CAD build for the part. Positions are in the model's coordinates, mm. A direction names the side the tool comes from. Give positions to 0.01 mm unless a question says otherwise; leave off trailing zeros. Loops run counter-clockwise (first coordinate to the right, second up) from the corner with the lowest first, then second, coordinate; pieces in that order, holes last. Notation, with made-up numbers: M 20.5,71.25 L 76.5,71.25 A20 ccw 76.5,94.25 Z; hole C 30,48.25 d1. An arc over 180 degrees is marked long. Answer as CSV lines item,"result".
```python
from build123d import *

# Parameters (mm, degrees)
BOSS_EXTRUDE1_DEPTH = 7
SKETCH2_R           = 5
CUT_EXTRUDE1_DEPTH  = 211.309296038
SKETCH3_R           = 2
CUT_EXTRUDE2_DEPTH  = 211.309296038


with BuildPart() as part:
    # Sketch1 → Boss-Extrude1 (new body)
    with BuildSketch(Plane(origin=(0, 0, 0), x_dir=(1, 0, 0), z_dir=(0, 1, 0))):
        with BuildLine():
            Line((6.708203932, 6), (53.291796068, 6))
            ThreePointArc((53.291796068, 6), (56.325765386, 8.215838363), (60, 9))
            Line((60, 9), (210, 9))
            Line((210, 9), (210, -9))
            Line((210, -9), (60, -9))
            ThreePointArc((60, -9), (56.325765386, -8.215838363), (53.291796068, -6))
            Line((53.291796068, -6), (6.708203932, -6))
            ThreePointArc((6.708203932, -6), (-9, 0), (6.708203932, 6))
        make_face()
    extrude(amount=BOSS_EXTRUDE1_DEPTH)

    # Sketch2 → Cut-Extrude1 (cut, through all)
    with BuildSketch(Plane(origin=(0, 7, 0), x_dir=(1, 0, 0), z_dir=(0, 1, 0))):
        with Locations(Location((0, 0, 0), (0, 0, 270))):
            Circle(SKETCH2_R)
        with Locations(Location((60, 0, 0), (0, 0, 270))):
            Circle(SKETCH2_R)
    extrude(amount=-CUT_EXTRUDE1_DEPTH, mode=Mode.SUBTRACT)

    # Sketch3 → Cut-Extrude2 (cut, through all)
    with BuildSketch(Plane(origin=(0, 7, 0), x_dir=(1, 0, 0), z_dir=(0, 1, 0))):
        with Locations(Location((200, 0, 0), (0, 0, 270))):
            Circle(SKETCH3_R)
        with Locations(Location((180, 0, 0), (0, 0, 270))):
            Circle(SKETCH3_R)
    extrude(amount=-CUT_EXTRUDE2_DEPTH, mode=Mode.SUBTRACT)


solid = part.part
```
Q1. Which spindle directions (+Z, -Z, +X, -X, +Y, -Y) get a long thin tool onto all of the face, cutting with end or side? Do faces 1 (the cylindrical face through (-9, 3, 0)), 2 (the flat face through (30, 3, -6)), 3 (the cylindrical face through (56.374, 3.451, 8.237)). Say none if no direction does.
Solution:
face 1,"+Y, -Y"
face 2,"-Z, +Y, -Y"
face 3,"+Z, +Y, -Y"
Q2. Cut at C-C (y = 4.75). Write the cut outline in (x, z), and give its area (3 significant figures).
Solution:
outline,"M 6.71,-6 L 53.29,-6 A9 ccw 60,-9 L 210,-9 L 210,9 L 60,9 A9 ccw 53.29,6 L 6.71,6 A9 ccw long Z; hole C 0,0 d10; hole C 60,0 d10; hole C 180,0 d4; hole C 200,0 d4"
area,"3,420 mm²"
Q3. Pin check, flat tips, straight feed: P1, Ø2.5, axis at x = 200, z = 0, coming from the -Y side; P2, Ø3.5, axis at x = 28, y = 5, coming from the +Z side; P3, Ø3, axis at y = 2, z = 3, coming from the -X side. Stop position of each tip, or through.
Solution:
P1,"passes through"
P2,"stops at z = 6"
P3,"stops at x = -8.87"
Q4. Cut at D-D (x = 180). Write the cut outline in (y, z).
Solution:
outline,"M 0,-9 L 7,-9 L 7,-2 L 0,-2 Z; M 0,2 L 7,2 L 7,9 L 0,9 Z"
Q5. Cut at A-A (x = 0). Write the cut outline in (y, z).
Solution:
outline,"M 0,-9 L 7,-9 L 7,-5 L 0,-5 Z; M 0,5 L 7,5 L 7,9 L 0,9 Z"
Q6. Cut at B-B (z = 0). Write the cut outline in (x, y), and give its area (3 significant figures).
Solution:
outline,"M -9,0 L -5,0 L -5,7 L -9,7 Z; M 5,0 L 55,0 L 55,7 L 5,7 Z; M 65,0 L 178,0 L 178,7 L 65,7 Z; M 182,0 L 198,0 L 198,7 L 182,7 Z; M 202,0 L 210,0 L 210,7 L 202,7 Z"
area,"1,340 mm²"
Q7. Wall check: line 1 (X direction, y = 4.75, z = 0); line 2 (Z direction, x = 200, y = 5.25); line 3 (X direction, y = 6.25, z = 2.25). Give the ranges that are in metal, low to high. Write a range as [from, to].
Solution:
line 1,"x = [-9, -5], [5, 55], [65, 178], [182, 198], [202, 210]"
line 2,"z = [-9, -2], [2, 9]"
line 3,"x = [-8.71, -4.47], [4.47, 55.53], [64.47, 210]"
